```python
from build123d import *

# Parameters (mm, degrees)
SKETCH_1_W      = 32
SKETCH_1_H      = 24
EXTRUDE_1_DEPTH = 4.5
SKETCH_2_R      = 9
SKETCH_2_W      = 4
SKETCH_2_H      = 12
EXTRUDE_2_DEPTH = 26
SKETCH_3_W      = 30
SKETCH_3_H      = 12
EXTRUDE_3_DEPTH = 4
SKETCH_4_R      = 0.4
EXTRUDE_4_DEPTH = 6


with BuildPart() as part:
    # 스케치1 → 보스-돌출1 (new body)
    with BuildSketch(Plane(origin=(0, 0, 0), x_dir=(1, 0, 0), z_dir=(0, 1, 0))):
        Rectangle(SKETCH_1_W, SKETCH_1_H)
    extrude(amount=EXTRUDE_1_DEPTH)

    # 스케치2 → 보스-돌출2 (add)
    with BuildSketch(Plane(origin=(0, 4.5, 0), x_dir=(1, 0, 0), z_dir=(0, 1, 0))):
        with Locations(Location((0, 0, 0), (0, 0, 90))):
            Circle(SKETCH_2_R)
        with Locations((-13, 0)):
            Rectangle(SKETCH_2_W, SKETCH_2_H)
        with Locations((13, 0)):
            Rectangle(SKETCH_2_W, SKETCH_2_H)
    extrude(amount=EXTRUDE_2_DEPTH)

    # 스케치3 → 보스-돌출3 (add)
    with BuildSketch(Plane(origin=(0, 30.5, 0), x_dir=(1, 0, 0), z_dir=(0, 1, 0))):
        Rectangle(SKETCH_3_W, SKETCH_3_H)
    extrude(amount=EXTRUDE_3_DEPTH)

    # 스케치4 → 보스-돌출4 (add)
    with BuildSketch(Plane.XZ):
        with Locations(Location((2.5, -8.75, 0), (0, 0, 90))):
            Circle(SKETCH_4_R)
        with Locations(Location((7.5, -8.75, 0), (0, 0, 90))):
            Circle(SKETCH_4_R)
        with Locations(Location((12.5, -8.75, 0), (0, 0, 90))):
            Circle(SKETCH_4_R)
        with Locations(Location((-12.5, -8.75, 0), (0, 0, 90))):
            Circle(SKETCH_4_R)
        with Locations(Location((-7.5, -8.75, 0), (0, 0, 90))):
            Circle(SKETCH_4_R)
        with Locations(Location((-2.5, -8.75, 0), (0, 0, 90))):
            Circle(SKETCH_4_R)
        with Locations(Location((-2.5, 8.75, 0), (0, 0, 90))):
            Circle(SKETCH_4_R)
        with Locations(Location((-7.5, 8.75, 0), (0, 0, 90))):
            Circle(SKETCH_4_R)
        with Locations(Location((-12.5, 8.75, 0), (0, 0, 90))):
            Circle(SKETCH_4_R)
        with Locations(Location((12.5, 8.75, 0), (0, 0, 90))):
            Circle(SKETCH_4_R)
        with Locations(Location((7.5, 8.75, 0), (0, 0, 90))):
            Circle(SKETCH_4_R)
        with Locations(Location((2.5, 8.75, 0), (0, 0, 90))):
            Circle(SKETCH_4_R)
    extrude(amount=EXTRUDE_4_DEPTH)


solid = part.part
```
Could you check a few things on this model? Use its own coordinates, in mm. A direction names the side the tool comes from. Coordinates: 2 decimals unless noted, no trailing zeros. Order: outer loops, then holes, each group sorted by start corner. A loop starts at its lowest first (then second) coordinate and runs counter-clockwise, first axis right, second up. Notation, with made-up numbers: M 67.5,-9.75 L 95.5,-9.75 A16 ccw 95.5,-5.75 Z; hole C 87.25,22 d5. An arc over 180 degrees is marked long. Use a Markdown table: item, result. Add a question column.
Q1. I want a section at A-A on y = 13. List the corners of the cut face in (x, z) for me, then the cut area to 3 significant figures.
Q2. I want a section at C-C on z = 0. List the corners of the cut face in (x, y) for me.
Q3. Which directions (+Z, -Z, +X, -X, +Y, -Y) give clear straight access to the entire face, cutting with the end or side of a thin tool? Please do faces 1 (the flat face through (0, 31, 6)), 2 (the flat face through (0, 30.5, -7)), 3 (the flat face through (0, 31, -6)), 4 (the flat face through (-7, 4.5, -6)), 5 (the flat face through (0, 30.5, 7)).
Q4. We'd pull the mould along X, two halves only. Please class faces 6 (the cylindrical face through (-2.703, 17.318, -8.584)), 7 (the flat face through (-11, 17, 0)), 8 (the flat face through (0, 2, 12)), 9 (the flat face through (-15, 19, 0)): pulls with the +X half, pulls with the -X half, needs draft (parallel to the pull), parting line crosses it, or undercut.
Q5. I want a section at B-B on x = 9.5. List the corners of the cut face in (y, z) for me, then the cut area to 3 significant figures.
Q6. If I drill on L1, parallel to Y at x = -9.5, z = -0.75; L2, parallel to X at y = 5, z = -3; L3, parallel to X at y = 5, z = 4, over which ranges is the centre line in solid material (lowest first)?
Q7. I'm going to push flat-ended pins straight in: pin 1 (2 mm diameter, centred on x = -9, y = 13.5, fed in from +Z); pin 2 (3 mm diameter, centred on x = 5, y = 6.5, fed in from +Z); pin 3 (3.5 mm diameter, centred on x = -1, z = -7.5, fed in from +Y); pin 4 (6 mm diameter, centred on y = 22.5, z = 3, fed in from +X). Where does each tip first touch, or does it pass through?
Q8. I want a section at D-D on y = -3.5. Give the number of separate pieces and of enclosed holes in the cut face, then the cut area to 3 significant figures.
Checked values:
| question | item | result |
|---|---|---|
| 1 | outline | M -15,-6 L -11,-6 L -11,6 L -15,6 Z; C 0,0 d18; M 11,-6 L 15,-6 L 15,6 L 11,6 Z |
| 1 | area | 350 mm² |
| 2 | outline | M -16,0 L 16,0 L 16,4.5 L 15,4.5 L 15,34.5 L -15,34.5 L -15,4.5 L -16,4.5 Z; hole M -11,4.5 L -9,4.5 L -9,30.5 L -11,30.5 Z; hole M 9,4.5 L 11,4.5 L 11,30.5 L 9,30.5 Z |
| 3 | face 1 | +Z, +Y |
| 3 | face 2 | -Z, +X, -X, +Y |
| 3 | face 3 | -Z, +Y |
| 3 | face 4 | none |
| 3 | face 5 | +Z, +X, -X, +Y |
| 4 | face 6 | undercut |
| 4 | face 7 | undercut |
| 4 | face 8 | needs draft |
| 4 | face 9 | pulls with the -X half |
| 5 | outline | M 0,-12 L 4.5,-12 L 4.5,12 L 0,12 Z; M 30.5,-6 L 34.5,-6 L 34.5,6 L 30.5,6 Z |
| 5 | area | 156 mm² |
| 6 | L1 | 0 to 4.5, 30.5 to 34.5 |
| 6 | L2 | -15 to -11, -8.49 to 8.49, 11 to 15 |
| 6 | L3 | -15 to -11, -8.06 to 8.06, 11 to 15 |
| 7 | pin 1 | z = 4.12 |
| 7 | pin 2 | z = 8.29 |
| 7 | pin 3 | y = 34.5 |
| 7 | pin 4 | x = 15 |
| 8 | separate pieces | 12 |
| 8 | enclosed holes | 0 |
| 8 | area | 6.03 mm² |
